Verification items for the finished model (mm, model axes). Coordinates: 2 decimals unless noted, no trailing zeros. Loops run counter-clockwise (first coordinate to the right, second up) from the corner with the lowest first, then second, coordinate; pieces in that order, holes last. Notation, with made-up numbers: (-14.5, 32) - (7.5, 32) arc R27 cw to (7.5, 57) - close; hole circle Ø4 at (29.25, -8.75). An arc over 180 degrees is marked (long way). Answer as CSV lines item,"result". Start each with the question number.
1. Cross-section at B-B (z = 0). Enter the section's corners in (x, y), plus the area to 3 significant figures.
2. Release check for a two-part mould opening along Y. For faces 1 (the cylindrical face through (12.81, -30.86, -43.16)), 2 (the cylindrical face through (12.878, -3.061, -13.785)), 3 (the flat face through (13, 0, -50.8)), 4 (the flat face through (13, 38.1, 0)) record: pulls with the +Y half, pulls with the -Y half, needs draft (parallel to the pull), parting line crosses it, or undercut.
3. Material ranges on line 1 (Z direction, x = 13.25, y = 0); line 2 (Z direction, x = 23, y = 5); line 3 (Y direction, x = 6.75, z = 9.5), recorded low to high. Write a range as [from, to].
4. Cross-section at D-D (x = 23.25). Enter the section's corners in (y, z), plus the area to 3 significant figures.
5. Cross-section at A-A (y = 0). Enter the section's corners in (x, z).
6. Cross-section at C-C (x = 17.25). Enter the section's corners in (y, z).
7. Gauge pin test, flat end, axial feed: P1, Ø3, axis at x = 7.5, y = -13.5, coming from the +Z side. Record the tip position at first contact, or that the pin passes through.
```python
from build123d import *

# Parameters (mm, degrees)
F0_W     = 76.2
F0_H     = 101.6
F1_DEPTH = 25.4
F2_R     = 14.120977
F3_DEPTH = 25.4
F4_R     = 25.4
F5_R     = 5.08


with BuildPart() as f1:
    # F0 (on Right) → F1 (new body)
    with BuildSketch(Plane.YZ):
        Rectangle(F0_W, F0_H)
    extrude(amount=F1_DEPTH)

    # F2 (on face) → F3 (cut)
    with BuildSketch(Plane.YZ.offset(25.4)):
        Circle(F2_R)
    extrude(amount=-F3_DEPTH, mode=Mode.SUBTRACT)

    # F4
    f4_edges = [f1.edges().sort_by_distance(p)[0] for p in [
        (12.7, -38.1, 50.8),
        (12.7, -38.1, -50.8),
        (12.7, 38.1, 50.8),
        (12.7, 38.1, -50.8),
    ]]
    fillet(f4_edges, radius=F4_R)

    # F5
    f5_edges = [f1.edges().sort_by_distance(p)[0] for p in [
        (25.4, 38.1, 0),
        (0, 38.1, 0),
    ]]
    fillet(f5_edges, radius=F5_R)


solid = f1.part
```
Values follow:
1,outline,"(0, -33.02) arc R5.08 ccw to (5.08, -38.1) - (20.32, -38.1) arc R5.08 ccw to (25.4, -33.02) - (25.4, -14.12) - (0, -14.12) - close; (0, 14.12) - (25.4, 14.12) - (25.4, 33.02) arc R5.08 ccw to (20.32, 38.1) - (5.08, 38.1) arc R5.08 ccw to (0, 33.02) - close"
1,area,"1,200 mm²"
2,face 1,"pulls with the -Y half"
2,face 2,"undercut"
2,face 3,"needs draft"
2,face 4,"pulls with the +Y half"
3,line 1,"z = [-50.8, -14.12], [14.12, 50.8]"
3,line 2,"z = [-50.04, -13.21], [13.21, 50.04]"
3,line 3,"y = [-38.1, -10.45], [10.45, 38.1]"
4,outline,"(-37.17, -25.4) arc R24.47 ccw to (-12.7, -49.87) - (12.7, -49.87) arc R24.47 ccw to (37.17, -25.4) - (37.17, 25.4) arc R24.47 ccw to (12.7, 49.87) - (-12.7, 49.87) arc R24.47 ccw to (-37.17, 25.4) - close; hole circle Ø28.24 at (0, 0)"
4,area,"6,270 mm²"
5,outline,"(0, -45.72) arc R5.08 ccw to (5.08, -50.8) - (20.32, -50.8) arc R5.08 ccw to (25.4, -45.72) - (25.4, -14.12) - (0, -14.12) - close; (0, 14.12) - (25.4, 14.12) - (25.4, 45.72) arc R5.08 ccw to (20.32, 50.8) - (5.08, 50.8) arc R5.08 ccw to (0, 45.72) - close"
6,outline,"(-38.1, -25.4) arc R25.4 ccw to (-12.7, -50.8) - (12.7, -50.8) arc R25.4 ccw to (38.1, -25.4) - (38.1, 25.4) arc R25.4 ccw to (12.7, 50.8) - (-12.7, 50.8) arc R25.4 ccw to (-38.1, 25.4) - close; hole circle Ø28.24 at (0, 0)"
7,P1,"stops at z = 50.8"
